Geometry: final body of the model. Coordinates: model frame, mm. Face numbers are marked on the shaded views. A direction names the side the tool comes from. Coordinates: 2 decimals unless noted, no trailing zeros. Loops run counter-clockwise (first coordinate to the right, second up) from the corner with the lowest first, then second, coordinate; pieces in that order, holes last. Notation, with made-up numbers: (-26, -22) - (-21, -22) arc R19 cw to (-21, -15) - close; hole circle Ø4 at (31, 51.25). An arc over 180 degrees is marked (long way). Put each result on its own line as item: value. Start each with the question number.
1) Material intervals for line 1 along X through (y, z) = (-2.5, -27); line 2 along Y through (x, z) = (29, -8.5); line 3 along X through (y, z) = (-3, 26.5), sorted ascending. Write a range as from..to.
2) Contact query for flat-ended pins moving along their axis: pin 1 Ø10.5 at (x, z) = (-13, 20.5) entering from -Y; pin 2 Ø14 at (x, z) = (12.5, 22.5) entering from -Y; pin 3 Ø4 at (y, z) = (-1, -9) entering from -X. Output: stop coordinate, or through.
3) Reachability of the marked faces 5, 6 and 7 from +Z, -Z, +X, -X, +Y, -Y: full face, straight path, thin tool, end or side. Return the list, or none.
4) Draft query along Z for the marked faces 1, 2, 3 and 4. Return one class per face: +Z half, -Z half, draft (parallel to the pull), parting line (faces both ways), or undercut.
5) Section C-C on x = 23. Output: boundary loops of the cut face in (y, z), and give its area (3 significant figures).
6) Section B-B on z = -25. Output: boundary loops of the cut face in (x, y).
```python
from build123d import *

# Parameters (mm, degrees)
F1_DEPTH = 6.35
F2_SIZE  = 2.54
F3_R     = 22.225
F4_DEPTH = 3.175
F5_SIZE2 = 2.54
F5_SIZE  = 3.81
F7_DEPTH = 2.54


with BuildPart() as f1:
    # F0 (on Front) → F1 (new body)
    with BuildSketch(Plane.XZ):
        with BuildLine():
            ThreePointArc((20.5490316571, -14.9297454082), (24.1568355139, -7.8490316571), (25.4, 0))
            ThreePointArc((25.4, 0), (24.1568355139, 7.8490316571), (20.5490316571, 14.9297454082))
            ThreePointArc((20.5490316571, 14.9297454082), (14.9297454082, 20.5490316571), (7.8490316571, 24.1568355139))
            ThreePointArc((7.8490316571, 24.1568355139), (0, 25.4), (-7.8490316571, 24.1568355139))
            ThreePointArc((-7.8490316571, 24.1568355139), (-14.9297454082, 20.5490316571), (-20.5490316571, 14.9297454082))
            ThreePointArc((-20.5490316571, 14.9297454082), (-24.1568355139, 7.8490316571), (-25.4, 0))
            ThreePointArc((-25.4, 0), (-24.1568355139, -7.8490316571), (-20.5490316571, -14.9297454082))
            ThreePointArc((-20.5490316571, -14.9297454082), (-14.9297454082, -20.5490316571), (-7.8490316571, -24.1568355139))
            ThreePointArc((-7.8490316571, -24.1568355139), (0, -25.4), (7.8490316571, -24.1568355139))
            ThreePointArc((7.8490316571, -24.1568355139), (14.9297454082, -20.5490316571), (20.5490316571, -14.9297454082))
        make_face()
        with BuildLine():
            Line((33.055969229, -4.6001704102), (25.4, 0))
            ThreePointArc((25.4, 0), (24.1568355139, -7.8490316571), (20.5490316571, -14.9297454082))
            Line((20.5490316571, -14.9297454082), (29.4467531969, -15.7081951742))
            Line((29.4467531969, -15.7081951742), (33.055969229, -4.6001704102))
        make_face()
        with BuildLine():
            ThreePointArc((20.5490316571, 14.9297454082), (24.1568355139, 7.8490316571), (25.4, 0))
            Line((25.4, 0), (33.055969229, 4.6001704102))
            Line((33.055969229, 4.6001704102), (29.4467531969, 15.7081951742))
            Line((29.4467531969, 15.7081951742), (20.5490316571, 14.9297454082))
        make_face()
        with BuildLine():
            ThreePointArc((7.8490316571, 24.1568355139), (14.9297454082, 20.5490316571), (20.5490316571, 14.9297454082))
            Line((20.5490316571, 14.9297454082), (24.0389285466, 23.1514272519))
            Line((24.0389285466, 23.1514272519), (14.589878302, 30.0165641039))
            Line((14.589878302, 30.0165641039), (7.8490316571, 24.1568355139))
        make_face()
        with BuildLine():
            Line((24.0389285466, -23.1514272519), (20.5490316571, -14.9297454082))
            ThreePointArc((20.5490316571, -14.9297454082), (14.9297454082, -20.5490316571), (7.8490316571, -24.1568355139))
            Line((7.8490316571, -24.1568355139), (14.589878302, -30.0165641039))
            Line((14.589878302, -30.0165641039), (24.0389285466, -23.1514272519))
        make_face()
        with BuildLine():
            ThreePointArc((-7.8490316571, 24.1568355139), (0, 25.4), (7.8490316571, 24.1568355139))
            Line((7.8490316571, 24.1568355139), (5.8398342126, 32.8596257714))
            Line((5.8398342126, 32.8596257714), (-5.8398342126, 32.8596257714))
            Line((-5.8398342126, 32.8596257714), (-7.8490316571, 24.1568355139))
        make_face()
        with BuildLine():
            Line((5.8398342126, -32.8596257714), (7.8490316571, -24.1568355139))
            ThreePointArc((7.8490316571, -24.1568355139), (0, -25.4), (-7.8490316571, -24.1568355139))
            Line((-7.8490316571, -24.1568355139), (-5.8398342126, -32.8596257714))
            Line((-5.8398342126, -32.8596257714), (5.8398342126, -32.8596257714))
        make_face()
        with BuildLine():
            ThreePointArc((-20.5490316571, 14.9297454082), (-14.9297454082, 20.5490316571), (-7.8490316571, 24.1568355139))
            Line((-7.8490316571, 24.1568355139), (-14.589878302, 30.0165641039))
            Line((-14.589878302, 30.0165641039), (-24.0389285466, 23.1514272519))
            Line((-24.0389285466, 23.1514272519), (-20.5490316571, 14.9297454082))
        make_face()
        with BuildLine():
            Line((-14.589878302, -30.0165641039), (-7.8490316571, -24.1568355139))
            ThreePointArc((-7.8490316571, -24.1568355139), (-14.9297454082, -20.5490316571), (-20.5490316571, -14.9297454082))
            Line((-20.5490316571, -14.9297454082), (-24.0389285466, -23.1514272519))
            Line((-24.0389285466, -23.1514272519), (-14.589878302, -30.0165641039))
        make_face()
        with BuildLine():
            ThreePointArc((-25.4, 0), (-24.1568355139, 7.8490316571), (-20.5490316571, 14.9297454082))
            Line((-20.5490316571, 14.9297454082), (-29.4467531969, 15.7081951742))
            Line((-29.4467531969, 15.7081951742), (-33.055969229, 4.6001704102))
            Line((-33.055969229, 4.6001704102), (-25.4, 0))
        make_face()
        with BuildLine():
            Line((-29.4467531969, -15.7081951742), (-20.5490316571, -14.9297454082))
            ThreePointArc((-20.5490316571, -14.9297454082), (-24.1568355139, -7.8490316571), (-25.4, 0))
            Line((-25.4, 0), (-33.055969229, -4.6001704102))
            Line((-33.055969229, -4.6001704102), (-29.4467531969, -15.7081951742))
        make_face()
    extrude(amount=F1_DEPTH)

    # F2
    f2_edges = [f1.edges().sort_by_distance(p)[0] for p in [
        (-22.29398, -6.35, -19.040586),
        (-19.314403, -6.35, -26.583996),
        (-11.219455, -6.35, -27.0867),
        (-6.844433, -6.35, -28.508231),
        (0, -6.35, -32.859626),
        (6.844433, -6.35, -28.508231),
        (11.219455, -6.35, -27.0867),
        (19.314403, -6.35, -26.583996),
        (22.29398, -6.35, -19.040586),
        (24.997892, -6.35, -15.31897),
        (31.251361, -6.35, -10.154183),
        (29.227985, -6.35, -2.300085),
        (29.227985, -6.35, 2.300085),
        (31.251361, -6.35, 10.154183),
        (24.997892, -6.35, 15.31897),
        (22.29398, -6.35, 19.040586),
        (19.314403, -6.35, 26.583996),
        (11.219455, -6.35, 27.0867),
        (6.844433, -6.35, 28.508231),
        (0, -6.35, 32.859626),
        (-6.844433, -6.35, 28.508231),
        (-11.219455, -6.35, 27.0867),
        (-19.314403, -6.35, 26.583996),
        (-22.29398, -6.35, 19.040586),
        (-24.997892, -6.35, 15.31897),
        (-31.251361, -6.35, 10.154183),
        (-29.227985, -6.35, 2.300085),
        (-29.227985, -6.35, -2.300085),
        (-31.251361, -6.35, -10.154183),
        (-24.997892, -6.35, -15.31897),
    ]]
    chamfer(f2_edges, length=F2_SIZE)

    # F3 (on face) → F4 (join, symmetric)
    with BuildSketch(Plane.XZ.offset(6.35)):
        Circle(F3_R)
    extrude(amount=F4_DEPTH, both=True)

    # F5
    f5_edges = [f1.edges().sort_by_distance(p)[0] for p in [
        (-22.225, -9.525, 0),
    ]]
    f5_side = f1.faces().sort_by_distance((0, -9.525, 0))[0]
    chamfer(f5_edges, length=F5_SIZE, length2=F5_SIZE2, reference=f5_side)

    # F6 (on face) → F7 (cut)
    with BuildSketch(Plane.XZ.offset(9.525)):
        with BuildLine():
            Line((-2.921, 4.6450305921), (-17.8195374743, 4.6450305921))
            ThreePointArc((-17.8195374743, 4.6450305921), (-15.4210632515, -10.0649407943), (-2.921, -18.1818586509))
            Line((-2.921, -18.1818586509), (-2.921, 4.6450305921))
        make_face()
        with BuildLine():
            ThreePointArc((15.1371864744, 10.4870305921), (0, 18.415), (-15.1371864744, 10.4870305921))
            Line((-15.1371864744, 10.4870305921), (15.1371864744, 10.4870305921))
        make_face()
        with BuildLine():
            Line((2.921, 4.6450305921), (2.921, -18.1818586509))
            ThreePointArc((2.921, -18.1818586509), (14.0161057359, -11.9440782399), (18.415, 0))
            ThreePointArc((18.415, 0), (18.2655277448, 2.3415211306), (17.8195374743, 4.6450305921))
            Line((17.8195374743, 4.6450305921), (2.921, 4.6450305921))
        make_face()
    extrude(amount=-F7_DEPTH, mode=Mode.SUBTRACT)


solid = f1.part
```
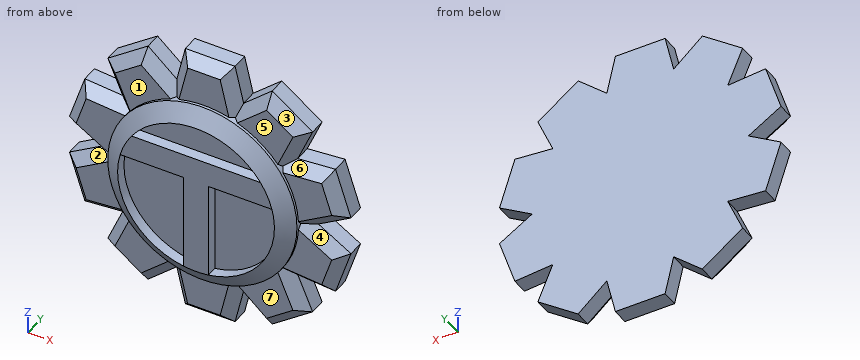
Answer block:
1. line 1: x = -18.74..-11.12, -7.19..7.19, 11.12..18.74
1. line 2: y = -6.35..0
1. line 3: x = -19.43..-10.54, -7.31..7.31, 10.54..19.43
2. pin 1: stops at y = -9.12
2. pin 2: stops at y = -9.31
2. pin 3: stops at x = -32.28
3. face 5: +Z, +X, -Y
3. face 6: -Y
3. face 7: -Z, +X, -Y
4. face 1: draft
4. face 2: undercut
4. face 3: +Z half
4. face 4: undercut
5. outline: (-6.35, -12.59) - (-3.81, -15.14) - (0, -15.14) - (0, 15.14) - (-3.81, 15.14) - (-6.35, 12.59) - (-6.35, 1.52) - (-5.05, 0) - (-6.35, -1.52) - close; (-4.65, -22.86) - (-3.81, -23.91) - (0, -23.91) - (0, -20.7) - (-3.81, -20.7) - close; (-4.65, 22.86) - (-3.81, 20.7) - (0, 20.7) - (0, 23.91) - (-3.81, 23.91) - close
5. area: 211 mm²
6. outline: (-21.49, -3.81) - (-17.17, -6.35) - (-12.69, -6.35) - (-8.82, -3.81) - (-8.82, 0) - (-21.49, 0) - close; (-7.65, -3.81) - (-5.05, -6.35) - (5.05, -6.35) - (7.65, -3.81) - (7.65, 0) - (-7.65, 0) - close; (8.82, -3.81) - (12.69, -6.35) - (17.17, -6.35) - (21.49, -3.81) - (21.49, 0) - (8.82, 0) - close
